Can you work these out from the model? Positions are in its coordinate system, mm. Face numbers are marked on the shaded views. A direction names the side the tool comes from. Coordinates: 2 decimals unless noted, no trailing zeros. Write each loop counter-clockwise with the first axis right and the second up, starting at its lowest first coordinate (ties: lowest second). Pieces come first, ordered by that corner, then holes. Notation, with made-up numbers: (70, -17) - (108, -17) arc R17 ccw to (108, 4) - close; hole circle Ø5 at (33, 59). An arc over 180 degrees is marked (long way). Use one line per item in the form item = value. Start each with the question number.
(1) If we section it at D-D on y = 10.5: Please give me the cut outline in (x, z).
(2) On a 3-axis mill with a long thin cutter (end or side, diameter ignored), from which of +Z, -Z, +X, -X, +Y, -Y can I reach the whole of each face in a straight line? I mean the marked faces 1 and 2. Say none if no direction works.
(3) For pin 1 Ø2.5 at (x, y) = (26, 13.5) entering from +Z; pin 2 Ø6 at (y, z) = (2, -22.5) entering from -X; pin 3 Ø2.5 at (x, y) = (28.5, 14) entering from -Z, each with a flat end and sliding along its axis, tell me the tip position at first contact or that it passes through.
(4) If we section it at A-A on x = 31: Please give me the cut outline in (y, z), then the cut area to 3 significant figures.
(5) If we section it at B-B on y = 5.75: Please give me the cut outline in (x, z), then the cut area to 3 significant figures.
(6) Thinking about a two-plate mould opening in X: for the marked faces 3, 4, 5 and 6, which applies, pulls with the +X half, pulls with the -X half, needs draft (parallel to the pull), parting line crosses it, or undercut?
(7) If we section it at C-C on x = 11.5: Please give me the cut outline in (y, z), then the cut area to 3 significant figures.
(8) If I drill on probe 1 along Z at (x, y) = (20, 8.75); probe 2 along Z at (x, y) = (29, 4.75); probe 3 along X at (y, z) = (7, -22.5), over which ranges is the centre line in solid material (lowest first)? Write a range as from..to.
```python
from build123d import *

# Parameters (mm, degrees)
BOSS_EXTRUDE1_DEPTH = 15
SKETCH2_4_W         = 49.5
SKETCH2_4_H         = 29.5
CUT_EXTRUDE1_DEPTH  = 7.5
SKETCH3_R           = 3
CUT_EXTRUDE2_DEPTH  = 6
SKETCH3_3_R         = 1.85
CUT_EXTRUDE3_DEPTH  = 16
SKETCH4_W           = 30
SKETCH4_H           = 12
CUT_EXTRUDE4_DEPTH  = 7.5
SKETCH4_3_W         = 36
SKETCH4_3_H         = 18
SKETCH4_3_W_2       = 30
SKETCH4_3_H_2       = 12
CUT_EXTRUDE5_DEPTH  = 3
FILLET2_R           = 3.5
SKETCH5_W           = 3
SKETCH5_H           = 30
CUT_EXTRUDE6_DEPTH  = 1.5


with BuildPart() as part:
    # Sketch2 → Boss-Extrude1 (new body)
    with BuildSketch(Plane(origin=(0, 0, 0), x_dir=(1, 0, 0), z_dir=(0, 1, 0))):
        with BuildLine():
            Line((9, 0), (62, 0))
            ThreePointArc((62, 0), (77.363961031, -6.363961031), (71, 9))
            Line((71, 9), (71, 31.5))
            ThreePointArc((71, 31.5), (77.363961031, 46.863961031), (62, 40.5))
            Line((62, 40.5), (9, 40.5))
            ThreePointArc((9, 40.5), (-6.363961031, 46.863961031), (0, 31.5))
            Line((0, 31.5), (0, 9))
            ThreePointArc((0, 9), (-6.363961031, -6.363961031), (9, 0))
        make_face()
    extrude(amount=BOSS_EXTRUDE1_DEPTH)

    # Sketch2<4> → Cut-Extrude1 (cut)
    with BuildSketch(Plane(origin=(0, 0, 0), x_dir=(1, 0, 0), z_dir=(0, 1, 0))):
        with Locations((32.75, 20.25)):
            Rectangle(SKETCH2_4_W, SKETCH2_4_H)
    extrude(amount=CUT_EXTRUDE1_DEPTH, mode=Mode.SUBTRACT)

    # Sketch3 → Cut-Extrude2 (cut)
    with BuildSketch(Plane(origin=(0, 15, 0), x_dir=(1, 0, 0), z_dir=(0, 1, 0))):
        Circle(SKETCH3_R)
        with Locations((0, 40.5)):
            Circle(SKETCH3_R)
        with Locations((71, 40.5)):
            Circle(SKETCH3_R)
        with Locations((71, 0)):
            Circle(SKETCH3_R)
    extrude(amount=-CUT_EXTRUDE2_DEPTH, mode=Mode.SUBTRACT)

    # Sketch3<3> → Cut-Extrude3 (cut, through all)
    with BuildSketch(Plane(origin=(0, 15, 0), x_dir=(1, 0, 0), z_dir=(0, 1, 0))):
        Circle(SKETCH3_3_R)
        with Locations((0, 40.5)):
            Circle(SKETCH3_3_R)
        with Locations((71, 40.5)):
            Circle(SKETCH3_3_R)
        with Locations((71, 0)):
            Circle(SKETCH3_3_R)
    extrude(amount=-CUT_EXTRUDE3_DEPTH, mode=Mode.SUBTRACT)

    # Sketch4 → Cut-Extrude4 (cut)
    with BuildSketch(Plane(origin=(0, 15, 0), x_dir=(1, 0, 0), z_dir=(0, 1, 0))):
        with Locations((33, 21)):
            Rectangle(SKETCH4_W, SKETCH4_H)
    extrude(amount=-CUT_EXTRUDE4_DEPTH, mode=Mode.SUBTRACT)

    # Sketch4<3> → Cut-Extrude5 (cut)
    with BuildSketch(Plane(origin=(0, 15, 0), x_dir=(1, 0, 0), z_dir=(0, 1, 0))):
        with Locations((33, 21)):
            Rectangle(SKETCH4_3_W, SKETCH4_3_H)
        with Locations((33, 21)):
            Rectangle(SKETCH4_3_W_2, SKETCH4_3_H_2, mode=Mode.SUBTRACT)
    extrude(amount=-CUT_EXTRUDE5_DEPTH, mode=Mode.SUBTRACT)

    # Fillet2
    fillet2_edges = [part.edges().sort_by_distance(p)[0] for p in [
        (77.363961031, 15, 6.363961031),
        (71, 15, -20.25),
        (77.363961031, 15, -46.863961031),
        (35.5, 15, -40.5),
        (-6.363961031, 15, -46.863961031),
        (0, 15, -20.25),
        (-6.363961031, 15, 6.363961031),
        (35.5, 15, 0),
    ]]
    fillet(fillet2_edges, radius=FILLET2_R)

    # Sketch5 → Cut-Extrude6 (cut)
    with BuildSketch(Plane.XZ):
        with Locations((66.5, -22)):
            Rectangle(SKETCH5_W, SKETCH5_H)
    extrude(amount=-CUT_EXTRUDE6_DEPTH, mode=Mode.SUBTRACT)


solid = part.part
```
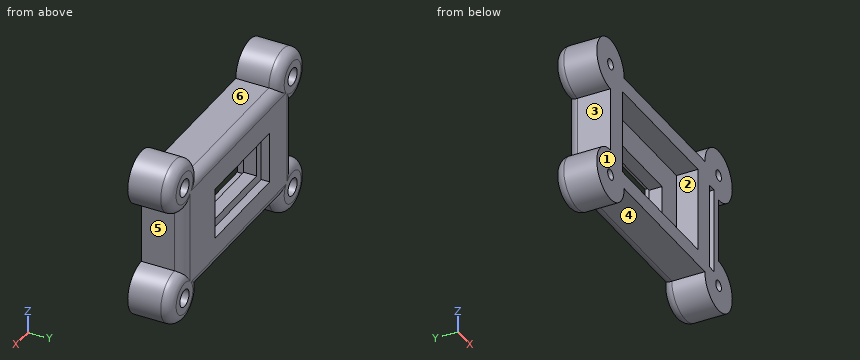
Reported:
q1.outline = (0, -31.5) arc R9 ccw (long way) to (9, -40.5) - (62, -40.5) arc R9 ccw (long way) to (71, -31.5) - (71, -9) arc R9 ccw (long way) to (62, 0) - (9, 0) arc R9 ccw (long way) to (0, -9) - close; hole circle Ø6 at (0, -40.5); hole circle Ø6 at (0, 0); hole (18, -27) - (48, -27) - (48, -15) - (18, -15) - close; hole circle Ø6 at (71, -40.5); hole circle Ø6 at (71, 0)
q2.face_1 = +Z, -Z, +X, -X, -Y
q2.face_2 = -Y
q3.pin_1 = -0.08
q3.pin_2 = 0
q3.pin_3 = -40.27
q4.outline = (0, -40.5) - (11.5, -40.5) arc R3.5 ccw to (15, -37) - (15, -30) - (12, -30) - (12, -27) - (7.5, -27) - (7.5, -35) - (0, -35) - close; (0, -5.5) - (7.5, -5.5) - (7.5, -15) - (12, -15) - (12, -12) - (15, -12) - (15, -3.5) arc R3.5 ccw to (11.5, 0) - (0, 0) - close
q4.area = 273 mm2
q5.outline = (0, -31.5) arc R9 ccw (long way) to (9, -40.5) - (62, -40.5) arc R9 ccw (long way) to (71, -31.5) - (71, -9) arc R9 ccw (long way) to (62, 0) - (9, 0) arc R9 ccw (long way) to (0, -9) - close; hole circle Ø3.7 at (0, -40.5); hole circle Ø3.7 at (0, 0); hole (8, -35) - (57.5, -35) - (57.5, -5.5) - (8, -5.5) - close; hole circle Ø3.7 at (71, -40.5); hole circle Ø3.7 at (71, 0)
q5.area = 2,140 mm2
q6.face_3 = pulls with the -X half
q6.face_4 = undercut
q6.face_5 = pulls with the +X half
q6.face_6 = undercut
q7.outline = (0, -40.5) - (11.5, -40.5) arc R3.5 ccw to (15, -37) - (15, -3.5) arc R3.5 ccw to (11.5, 0) - (0, 0) - (0, -5.5) - (7.5, -5.5) - (7.5, -35) - (0, -35) - close
q7.area = 381 mm2
q8.probe_1 = -40.5..-27, -15..0
q8.probe_2 = -40.5..-35, -5.5..0
q8.probe_3 = 0..8, 57.5..71
